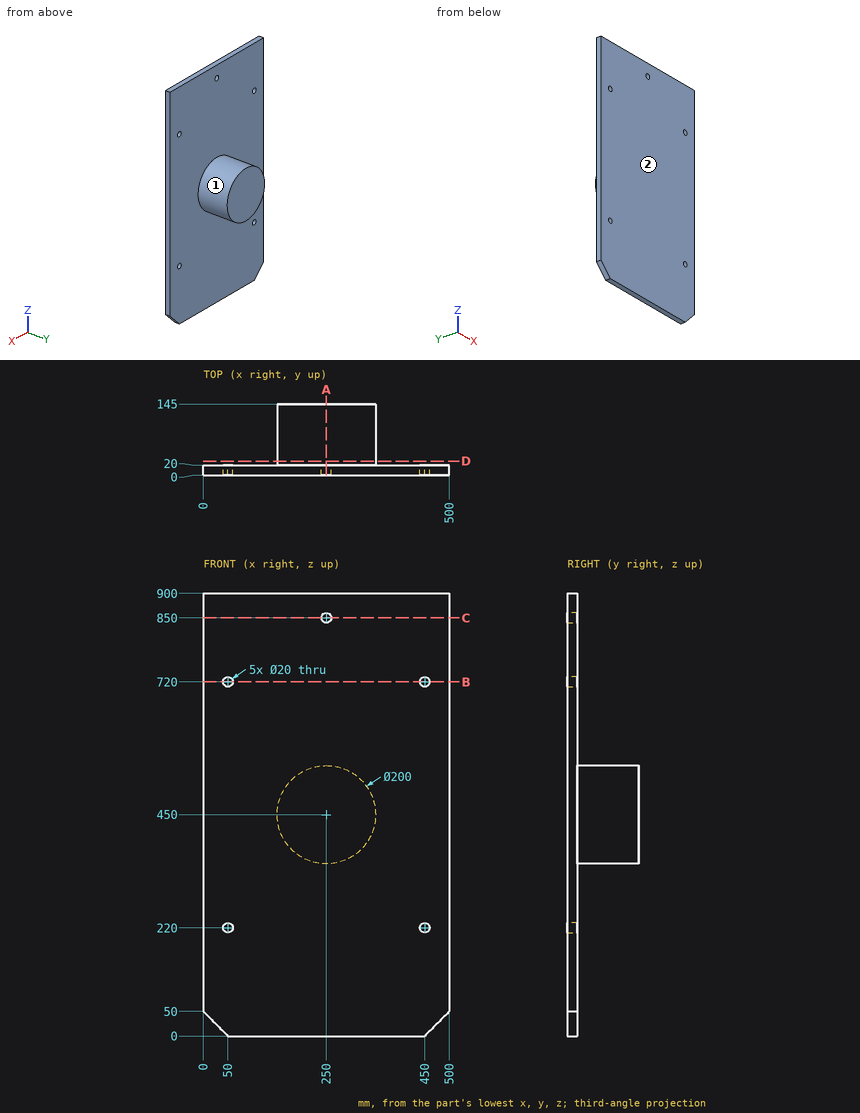
The figure shows three views and two pictorial views of one solid part (mm, origin at its lowest corner). Answer the questions. A direction names the side the tool comes from. Coordinates: 2 decimals unless noted, no trailing zeros. Write each loop counter-clockwise with the first axis right and the second up, starting at its lowest first coordinate (ties: lowest second). Pieces come first, ordered by that corner, then holes. Notation, with made-up numbers: (-20, 88) -> (21, 88) arc R17 cw to (21, 101) -> close; hole circle Ø5 at (86, 81.25). An arc over 180 degrees is marked (long way). Return JSON: item names as keys, results as strings.
(1) The part is cut by section D-D on y = 29. Give the vertices of the cut face in (x, z), then the cut area to 3 significant figures.
Answers below:
{"outline": "circle Ø200 at (250, 450)", "area": "31,400 mm^2"}
(2) Which of the six approach directions +Z, -Z, +X, -X, +Y, -Y give full straight-line access (tool end or side, diameter ignored) to the marked faces 1 and 2?
Answers below:
{"face 1": "+Y", "face 2": "+Z, -Z, +X, -X, -Y"}
(3) The part is cut by section B-B on z = 720. Give the vertices of the cut face in (x, y), then the cut area to 3 significant figures.
Answers below:
{"outline": "(0, 0) -> (40, 0) -> (40, 20) -> (0, 20) -> close; (60, 0) -> (440, 0) -> (440, 20) -> (60, 20) -> close; (460, 0) -> (500, 0) -> (500, 20) -> (460, 20) -> close", "area": "9,200 mm^2"}
(4) Each of these flat-tipped pins is pushed along its axis until it touches: P1, Ø3, axis at x = 264, y = 79.5, coming from the -Z side; P2, Ø1, axis at x = 329, z = 240.5, coming from the +Y side; P3, Ø12, axis at x = 450, z = 220, coming from the -Y side. Where does it stop, or does it pass through?
Answers below:
{"P1": "z = 350.78", "P2": "y = 20", "P3": "through"}
(5) The part is cut by section C-C on z = 850. Give the vertices of the cut face in (x, y), then the cut area to 3 significant figures.
Answers below:
{"outline": "(0, 0) -> (240, 0) -> (240, 20) -> (0, 20) -> close; (260, 0) -> (500, 0) -> (500, 20) -> (260, 20) -> close", "area": "9,600 mm^2"}
(6) Consider line 1 along X through (y, z) = (5.5, 720); line 2 along Y through (x, z) = (41.5, 401); line 3 along Z through (x, y) = (190.5, 61). Determine where each line is inside the solid, lowest interval first. Write a range as from..to.
Answers below:
{"line 1": "0..40, 60..440, 460..500", "line 2": "0..20", "line 3": "369.63..530.37"}
(7) The part is cut by section A-A on x = 250. Give the vertices of the cut face in (y, z).
Answers below:
{"outline": "(0, 0) -> (20, 0) -> (20, 350) -> (145, 350) -> (145, 550) -> (20, 550) -> (20, 840) -> (0, 840) -> close; (0, 860) -> (20, 860) -> (20, 900) -> (0, 900) -> close"}
